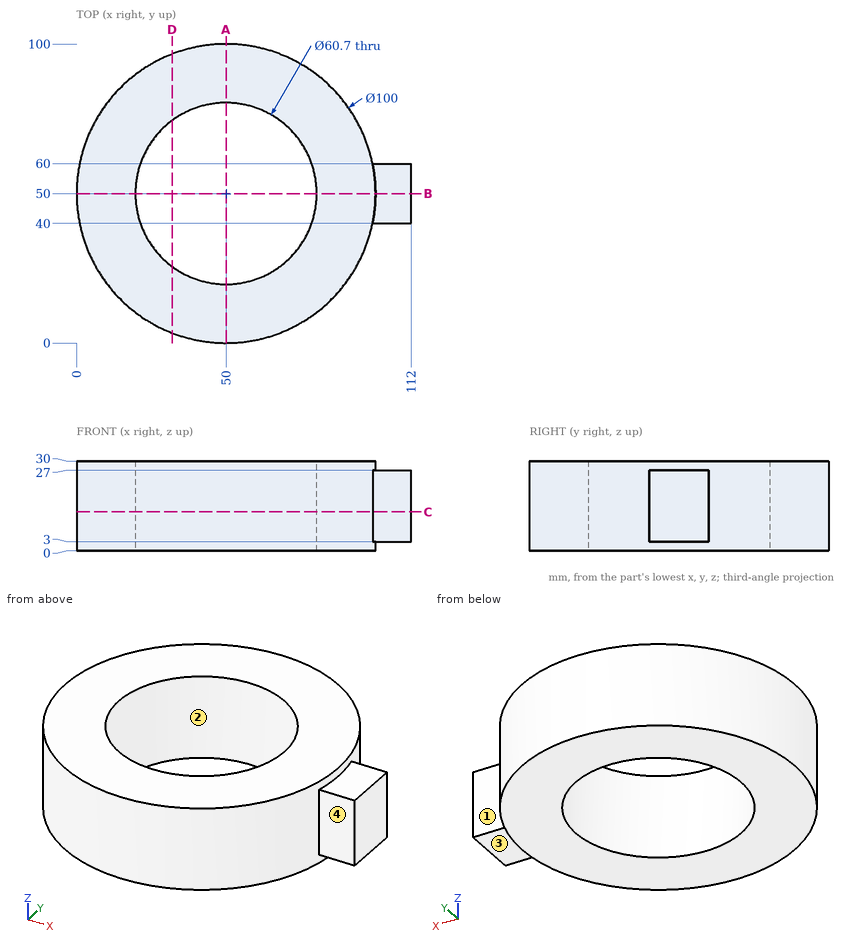
Job drawing, mm, ordinate dimensions from the low corner. One solid piece. Coordinates: 2 decimals unless noted, no trailing zeros. Order: outer loops, then holes, each group sorted by start corner. A loop starts at its lowest first (then second) coordinate and runs counter-clockwise, first axis right, second up. Notation, with made-up numbers: (51.5, 69.5) -> (78.5, 69.5) arc R5 ccw to (78.5, 77.5) -> close; hole circle Ø8 at (71, 80.25). An arc over 180 degrees is marked (long way). Answer in a Markdown table with one row per item. Add a question column.
Q1. Band-saw the part on D-D, the plane x = 32. List the corners of the cut face in (y, z).
Q2. Drop flat-ended pins along their axis: pin 1 (5 mm diameter, centred on x = 30, z = 10, fed in from -Y); pin 2 (4 mm diameter, centred on y = 40.5, z = 19, fed in from -X); pin 3 (3 mm diameter, centred on x = 39, z = 17.5, fed in from +Y). Give the stop position or say it passes through.
Q3. Band-saw the part on A-A, the plane x = 50. List the corners of the cut face in (y, z).
Q4. Mould opens along Y. For the marked faces 1, 2, 3 and 4 say: +Y half, -Y half, draft (parallel to the pull), parting line (faces both ways), or undercut.
Q5. Band-saw the part on C-C, the plane z = 13. List the corners of the cut face in (x, y), then the cut area to 3 significant figures.
Q6. Band-saw the part on B-B, the plane y = 50. List the corners of the cut face in (x, z).
Q7. Wall check: line 1 along Y through (x, z) = (50, 12.25); line 2 along Y through (x, z) = (26.5, 4); line 3 along X through (y, z) = (45, 28.25). Give the ranges that are in metal, low to high. Write a range as [from, to].
Answers follow:
| question | item | result |
|---|---|---|
| 1 | outline | (3.35, 0) -> (25.56, 0) -> (25.56, 30) -> (3.35, 30) -> close; (74.44, 0) -> (96.65, 0) -> (96.65, 30) -> (74.44, 30) -> close |
| 2 | pin 1 | y = 3.16 |
| 2 | pin 2 | x = 0.57 |
| 2 | pin 3 | y = 99.09 |
| 3 | outline | (0, 0) -> (19.65, 0) -> (19.65, 30) -> (0, 30) -> close; (80.35, 0) -> (100, 0) -> (100, 30) -> (80.35, 30) -> close |
| 4 | face 1 | +Y half |
| 4 | face 2 | undercut |
| 4 | face 3 | draft |
| 4 | face 4 | -Y half |
| 5 | outline | (98.99, 40) -> (112, 40) -> (112, 60) -> (98.99, 60) arc R50 ccw (long way) to start; hole circle Ø60.7 at (50, 50) |
| 5 | area | 5,210 mm^2 |
| 6 | outline | (0, 0) -> (19.65, 0) -> (19.65, 30) -> (0, 30) -> close; (80.35, 0) -> (100, 0) -> (100, 3) -> (112, 3) -> (112, 27) -> (100, 27) -> (100, 30) -> (80.35, 30) -> close |
| 7 | line 1 | [0, 19.65], [80.35, 100] |
| 7 | line 2 | [5.87, 30.79], [69.21, 94.13] |
| 7 | line 3 | [0.25, 20.06], [79.94, 99.75] |
